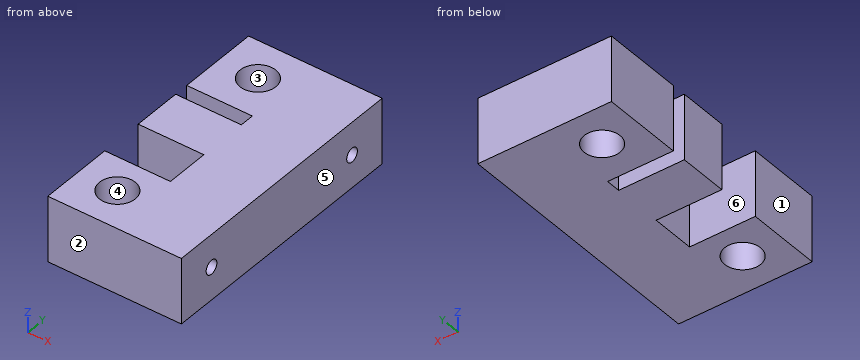
```python
from build123d import *

# Parameters (mm, degrees)
SKETCH1_W           = 30.5
SKETCH1_H           = 15
BOSS_EXTRUDE1_DEPTH = 60
SKETCH2_R           = 4.1
CUT_EXTRUDE1_DEPTH  = 16
SKETCH4_W           = 15
SKETCH4_H           = 3.3
CUT_EXTRUDE2_DEPTH  = 16
SKETCH5_W           = 15
SKETCH5_H           = 10
CUT_EXTRUDE3_DEPTH  = 16
SKETCH6_R           = 1.6
CUT_EXTRUDE4_DEPTH  = 15


with BuildPart() as part:
    # Sketch1 → Boss-Extrude1 (new body)
    with BuildSketch(Plane(origin=(0, 0, 0), x_dir=(1, 0, 0), z_dir=(0, 1, 0))):
        Rectangle(SKETCH1_W, SKETCH1_H)
    extrude(amount=BOSS_EXTRUDE1_DEPTH)

    # Sketch2 → Cut-Extrude1 (cut, through all)
    with BuildSketch(Plane.XY.offset(7.5)):
        with Locations((-6.25, 51)):
            Circle(SKETCH2_R)
        with Locations((-6.25, 9)):
            Circle(SKETCH2_R)
    extrude(amount=-CUT_EXTRUDE1_DEPTH, mode=Mode.SUBTRACT)

    # Sketch4 → Cut-Extrude2 (cut, through all)
    with BuildSketch(Plane.XY.offset(7.5)):
        with Locations((-7.75, 39.85)):
            Rectangle(SKETCH4_W, SKETCH4_H)
    extrude(amount=-CUT_EXTRUDE2_DEPTH, mode=Mode.SUBTRACT)

    # Sketch5 → Cut-Extrude3 (cut, through all)
    with BuildSketch(Plane.XY.offset(7.5)):
        with Locations((-7.75, 22)):
            Rectangle(SKETCH5_W, SKETCH5_H)
    extrude(amount=-CUT_EXTRUDE3_DEPTH, mode=Mode.SUBTRACT)

    # Sketch6 → Cut-Extrude4 (cut)
    with BuildSketch(Plane(origin=(15.25, 0, 0), x_dir=(0, 0, -1), z_dir=(1, 0, 0))):
        with Locations((0, 51)):
            Circle(SKETCH6_R)
        with Locations((0, 9)):
            Circle(SKETCH6_R)
    extrude(amount=-CUT_EXTRUDE4_DEPTH, mode=Mode.SUBTRACT)


solid = part.part
```
Verification items for the finished model (mm, model axes). Face numbers are marked on the shaded views. A direction names the side the tool comes from. Coordinates: 2 decimals unless noted, no trailing zeros. Order: outer loops, then holes, each group sorted by start corner. A loop starts at its lowest first (then second) coordinate and runs counter-clockwise, first axis right, second up. Notation, with made-up numbers: (-14, 81.25) -> (5, 81.25) arc R23 cw to (5, 98.25) -> close; hole circle Ø6 at (85.25, 69). An arc over 180 degrees is marked (long way). Answer as CSV lines item,"result". Start each with the question number.
1) Material ranges on L1, parallel to Y at x = -11, z = 6.25; L2, parallel to Y at x = -6.25, z = 3.5; L3, parallel to Y at x = 8.25, z = 0, recorded low to high. Write a range as [from, to].
2) Cross-section at C-C, the plane x = -6. Record the boundary of the cut face in (y, z), then the cut area to 3 significant figures.
3) Release check for a two-part mould opening along Y. For the marked faces 1, 2, 3 and 4 record: released by +Y, released by -Y, zero draft, split by the parting line, or undercut.
4) Cross-section at A-A, the plane z = 4. Record the boundary of the cut face in (x, y).
5) Cross-section at D-D, the plane x = 3.5. Record the boundary of the cut face in (y, z).
6) Gauge pin test, flat ends, axial feed: pin 1 Ø5 at (x, y) = (-6.25, 9) entering from +Z; pin 2 Ø5 at (y, z) = (23.5, -3) entering from -X. Record the tip position at first contact, or that the pin passes through.
7) Set-up check for the marked faces 5 and 6: record each of +Z, -Z, +X, -X, +Y, -Y from which the full face is reachable in a straight line by a thin tool's end or side.
8) Cross-section at B-B, the plane y = 51. Record the boundary of the cut face in (x, z), then the cut area to 4 significant figures.
Conclusion:
1,L1,"y = [0, 17], [27, 38.2], [41.5, 60]"
1,L2,"y = [0, 4.9], [13.1, 17], [27, 38.2], [41.5, 46.9], [55.1, 60]"
1,L3,"y = [0, 7.4], [10.6, 49.4], [52.6, 60]"
2,outline,"(0, -7.5) -> (4.91, -7.5) -> (4.91, 7.5) -> (0, 7.5) -> close; (13.09, -7.5) -> (17, -7.5) -> (17, 7.5) -> (13.09, 7.5) -> close; (27, -7.5) -> (38.2, -7.5) -> (38.2, 7.5) -> (27, 7.5) -> close; (41.5, -7.5) -> (46.91, -7.5) -> (46.91, 7.5) -> (41.5, 7.5) -> close; (55.09, -7.5) -> (60, -7.5) -> (60, 7.5) -> (55.09, 7.5) -> close"
2,area,"455 mm²"
3,face 1,"zero draft"
3,face 2,"released by -Y"
3,face 3,"undercut"
3,face 4,"undercut"
4,outline,"(-15.25, 0) -> (15.25, 0) -> (15.25, 60) -> (-15.25, 60) -> (-15.25, 41.5) -> (-0.25, 41.5) -> (-0.25, 38.2) -> (-15.25, 38.2) -> (-15.25, 27) -> (-0.25, 27) -> (-0.25, 17) -> (-15.25, 17) -> close; hole circle Ø8.2 at (-6.25, 9); hole circle Ø8.2 at (-6.25, 51)"
5,outline,"(0, -7.5) -> (60, -7.5) -> (60, 7.5) -> (0, 7.5) -> close; hole circle Ø3.2 at (9, 0); hole circle Ø3.2 at (51, 0)"
6,pin 1,"passes through"
6,pin 2,"stops at x = -0.25"
7,face 5,"+Z, -Z, +X, +Y, -Y"
7,face 6,"+Z, -Z, -X"
8,outline,"(-15.25, -7.5) -> (-10.35, -7.5) -> (-10.35, 7.5) -> (-15.25, 7.5) -> close; (-2.15, -7.5) -> (15.25, -7.5) -> (15.25, -1.6) -> (0.25, -1.6) -> (0.25, 1.6) -> (15.25, 1.6) -> (15.25, 7.5) -> (-2.15, 7.5) -> close"
8,area,"286.5 mm²"
